Could you check a few things on this model? Use its own coordinates, in mm. A direction names the side the tool comes from. Give positions to 0.01 mm unless a question says otherwise; leave off trailing zeros. Write each loop counter-clockwise with the first axis right and the second up, starting at its lowest first coordinate (ties: lowest second). Pieces come first, ordered by that corner, then holes. Notation, with made-up numbers: (48, -20.75) - (79, -20.75) arc R14 ccw to (79, -4.75) - close; hole circle Ø7 at (10.25, -13.5). An arc over 180 degrees is marked (long way). Use one line per item in the form item = value.
```python
from build123d import *

# Parameters (mm, degrees)
SKETCH1_W           = 100
SKETCH1_H           = 64
SKETCH1_R           = 1.95
BOSS_EXTRUDE1_DEPTH = 2
SKETCH2_R           = 5
SKETCH2_R_2         = 1.95
BOSS_EXTRUDE2_DEPTH = 5
SKETCH3_R           = 4.5
SKETCH3_R_2         = 1.425
BOSS_EXTRUDE3_DEPTH = 13
CUT_EXTRUDE1_DEPTH  = 120.436175424
FILLET1_R           = 5


with BuildPart() as part:
    # Sketch1 → Boss-Extrude1 (new body)
    with BuildSketch(Plane(origin=(0, 0, 0), x_dir=(0, 1, 0), z_dir=(0, 0, 1))):
        with Locations((50, 32)):
            Rectangle(SKETCH1_W, SKETCH1_H)
        with Locations(Location((90, 32, 0), (0, 0, 270))):
            Circle(SKETCH1_R, mode=Mode.SUBTRACT)
        with Locations(Location((50, 32, 0), (0, 0, 270))):
            Circle(SKETCH1_R, mode=Mode.SUBTRACT)
    extrude(amount=BOSS_EXTRUDE1_DEPTH)

    # Sketch2 → Boss-Extrude2 (add)
    # profile 1 of 2: a face of its own
    with BuildSketch(Plane.XY.offset(2)):
        with Locations((-32, 50)):
            Circle(SKETCH2_R)
        with Locations((-32, 50)):
            Circle(SKETCH2_R_2, mode=Mode.SUBTRACT)
    # profile 2 of 2: a face of its own
    with BuildSketch(Plane.XY.offset(2)):
        with Locations((-32, 90)):
            Circle(SKETCH2_R)
        with Locations((-32, 90)):
            Circle(SKETCH2_R_2, mode=Mode.SUBTRACT)
    extrude(amount=BOSS_EXTRUDE2_DEPTH)

    # Sketch3 → Boss-Extrude3 (add)
    # profile 1 of 4: a face of its own
    with BuildSketch(Plane.XY.offset(2)):
        with Locations(Location((-59, 5, 0), (0, 0, 180))):
            Circle(SKETCH3_R)
        with Locations(Location((-59, 5, 0), (0, 0, 180))):
            Circle(SKETCH3_R_2, mode=Mode.SUBTRACT)
    # profile 2 of 4: a face of its own
    with BuildSketch(Plane.XY.offset(2)):
        with Locations(Location((-5, 5, 0), (0, 0, 180))):
            Circle(SKETCH3_R)
        with Locations(Location((-5, 5, 0), (0, 0, 180))):
            Circle(SKETCH3_R_2, mode=Mode.SUBTRACT)
    # profile 3 of 4: a face of its own
    with BuildSketch(Plane.XY.offset(2)):
        with Locations(Location((-5, 52, 0), (0, 0, 180))):
            Circle(SKETCH3_R)
        with Locations(Location((-5, 52, 0), (0, 0, 180))):
            Circle(SKETCH3_R_2, mode=Mode.SUBTRACT)
    # profile 4 of 4: a face of its own
    with BuildSketch(Plane.XY.offset(2)):
        with Locations(Location((-59, 52, 0), (0, 0, 180))):
            Circle(SKETCH3_R)
        with Locations(Location((-59, 52, 0), (0, 0, 180))):
            Circle(SKETCH3_R_2, mode=Mode.SUBTRACT)
    extrude(amount=BOSS_EXTRUDE3_DEPTH)

    # Sketch4 → Cut-Extrude1 (cut, through all)
    with BuildSketch(Plane.XY.offset(2)):
        Polygon((-64, 100), (-36, 100), (-64, 60), align=None)
        Polygon((-28, 100), (0, 100), (0, 60), align=None)
    extrude(amount=-CUT_EXTRUDE1_DEPTH, mode=Mode.SUBTRACT)

    # Fillet1
    fillet1_edges = [part.edges().sort_by_distance(p)[0] for p in [
        (-64, 60, 1),
        (-36, 100, 1),
        (-64, 0, 1),
        (0, 60, 1),
        (-28, 100, 1),
        (0, 0, 1),
    ]]
    fillet(fillet1_edges, radius=FILLET1_R)


solid = part.part
```
1. Imagine slicing it at D-D, the plane y = 63.5. List the corners of the cut face in (x, z) for me, and give its area (3 significant figures).
Response values:
outline = (-61.55, 0) - (-2.45, 0) - (-2.45, 2) - (-61.55, 2) - close
area = 118 mm²
2. Which directions (+Z, -Z, +X, -X, +Y, -Y) give clear straight access to the entire face, cutting with the end or side of a thin tool? Please do faces 4 (the face through (-29.8, 50.1, 7)), 5 (the face through (-29.8, 90.1, 7)), 6 (the face through (-3.95, 4.037, 8.409)).
Response values:
face_4 = +Z, +Y, -Y
face_5 = +Z, +X, -X, +Y, -Y
face_6 = +Z
3. If I drill on line 1 (X direction, y = 52, z = 10.5) (3 decimals); line 2 (Y direction, x = -32, z = 4.75); line 3 (X direction, y = 52, z = 6.25) (3 decimals), over which ranges is the centre line in solid material (lowest first)? Write a range as from..to.
Response values:
line_1 = -63.5..-60.425, -57.575..-54.5, -9.5..-6.425, -3.575..-0.5
line_2 = 45..48.05, 51.95..55, 85..88.05, 91.95..95
line_3 = -63.5..-60.425, -57.575..-54.5, -36.583..-27.417, -9.5..-6.425, -3.575..-0.5
4. Imagine slicing it at A-A, the plane z = 10. List the corners of the cut face in (x, y) for me (3 decimals).
Response values:
outline = circle Ø9 at (-59, 5); circle Ø9 at (-59, 52); circle Ø9 at (-5, 5); circle Ø9 at (-5, 52); hole circle Ø2.85 at (-59, 5); hole circle Ø2.85 at (-59, 52); hole circle Ø2.85 at (-5, 5); hole circle Ø2.85 at (-5, 52)
5. Imagine slicing it at C-C, the plane x = -50. List the corners of the cut face in (y, z) for me.
Response values:
outline = (0, 0) - (80, 0) - (80, 2) - (0, 2) - close
6. Imagine slicing it at B-B, the plane y = 90. List the corners of the cut face in (x, z) for me, and give its area (3 significant figures).
Response values:
outline = (-43, 0) - (-33.95, 0) - (-33.95, 7) - (-37, 7) - (-37, 2) - (-43, 2) - close; (-30.05, 0) - (-21, 0) - (-21, 2) - (-27, 2) - (-27, 7) - (-30.05, 7) - close
area = 66.7 mm²
7. If we mould it in two halves opening along Y, with no side actions, what happens to faces 1 (the face through (-36, 53, 4)), 2 (the face through (-64, 31, 1)), 3 (the face through (-63.775, 59.907, 0.986))? For each: pulls with the +Y half, pulls with the -Y half, needs draft (parallel to the pull), parting line crosses it, or undercut.
Response values:
face_1 = undercut
face_2 = needs draft
face_3 = pulls with the +Y half
8. For pin 1 (4 mm diameter, centred on x = -50.5, y = 32.5, fed in from -Z); pin 2 (3 mm diameter, centred on x = -32, y = 90, fed in from +Z); pin 3 (4 mm diameter, centred on x = -42, y = 87, fed in from +Z); pin 4 (2 mm diameter, centred on x = -54.5, z = 11, fed in from +Y), each with a flat end and sliding along its axis, tell me the tip position at first contact or that it passes through.
Response values:
pin_1 = 0
pin_2 = through
pin_3 = 2
pin_4 = 54.83
